```python
from build123d import *

# Parameters (mm, degrees)
BOSS_EXTRUDE1_DEPTH = 3.175
SKETCH3_R           = 1.5
CUT_EXTRUDE2_DEPTH  = 112.800002795


with BuildPart() as part:
    # Sketch1 → Boss-Extrude1 (new body)
    with BuildSketch(Plane(origin=(0, 0, 0), x_dir=(1, 0, 0), z_dir=(0, 1, 0))):
        with BuildLine():
            ThreePointArc((59, 25.4), (57.242640687, 21.157359313), (53, 19.4))
            Line((53, 19.4), (53, 17.4))
            Line((53, 17.4), (53, 17))
            Line((53, 17), (74, 17))
            Line((74, 17), (91, 17))
            ThreePointArc((91, 17), (99.746427842, 14.577379737), (106, 8))
            Line((106, 8), (106, 35.4))
            Line((106, 35.4), (53, 35.4))
            Line((53, 35.4), (53, 31.4))
            ThreePointArc((53, 31.4), (57.242640687, 29.642640687), (59, 25.4))
        make_face()
        with BuildLine():
            ThreePointArc((106, 8), (99.746427842, 14.577379737), (91, 17))
            Line((91, 17), (91, 0))
            Line((91, 0), (106, 0))
            Line((106, 0), (106, 8))
        make_face()
        with BuildLine():
            Line((91, 0), (91, 17))
            ThreePointArc((91, 17), (86.600076233, 16.420739047), (82.5, 14.722431864))
            ThreePointArc((82.5, 14.722431864), (88.722431864, 8.5), (91, 0))
        make_face()
        with BuildLine():
            Line((91, 17), (74, 17))
            ThreePointArc((74, 17), (78.399923767, 16.420739047), (82.5, 14.722431864))
            ThreePointArc((82.5, 14.722431864), (86.600076233, 16.420739047), (91, 17))
        make_face()
        with BuildLine():
            Line((53, 17.4), (53, 19.4))
            ThreePointArc((53, 19.4), (47, 25.4), (53, 31.4))
            Line((53, 31.4), (53, 35.4))
            Line((53, 35.4), (0, 35.4))
            Line((0, 35.4), (0, 8))
            ThreePointArc((0, 8), (6.253572158, 14.577379737), (15, 17))
            Line((15, 17), (32, 17))
            Line((32, 17), (53, 17))
            Line((53, 17), (53, 17.4))
        make_face()
        with BuildLine():
            Line((15, 0), (15, 17))
            ThreePointArc((15, 17), (6.253572158, 14.577379737), (0, 8))
            Line((0, 8), (0, 0))
            Line((0, 0), (15, 0))
        make_face()
        with BuildLine():
            ThreePointArc((23.5, 14.722431864), (19.399923767, 16.420739047), (15, 17))
            Line((15, 17), (15, 0))
            ThreePointArc((15, 0), (17.277568136, 8.5), (23.5, 14.722431864))
        make_face()
        with BuildLine():
            ThreePointArc((23.5, 14.722431864), (27.600076233, 16.420739047), (32, 17))
            Line((32, 17), (15, 17))
            ThreePointArc((15, 17), (19.399923767, 16.420739047), (23.5, 14.722431864))
        make_face()
    extrude(amount=BOSS_EXTRUDE1_DEPTH)

    # Sketch3 → Cut-Extrude2 (cut, through all)
    with BuildSketch(Plane.XZ):
        with BuildLine():
            ThreePointArc((9, -15), (8.560660172, -13.939339828), (7.5, -13.5))
            Line((7.5, -13.5), (7.5, -16.5))
            ThreePointArc((7.5, -16.5), (8.560660172, -16.060660172), (9, -15))
        make_face()
        with BuildLine():
            Line((7.5, -16.5), (7.5, -13.5))
            ThreePointArc((7.5, -13.5), (6, -15), (7.5, -16.5))
        make_face()
        with Locations(Location((98.5, -15, 0), (0, 0, 270))):
            Circle(SKETCH3_R)
        with Locations(Location((98.5, -7.5, 0), (0, 0, 270))):
            Circle(SKETCH3_R)
        with Locations(Location((7.5, -7.5, 0), (0, 0, 270))):
            Circle(SKETCH3_R)
    extrude(amount=-CUT_EXTRUDE2_DEPTH, mode=Mode.SUBTRACT)


solid = part.part
```
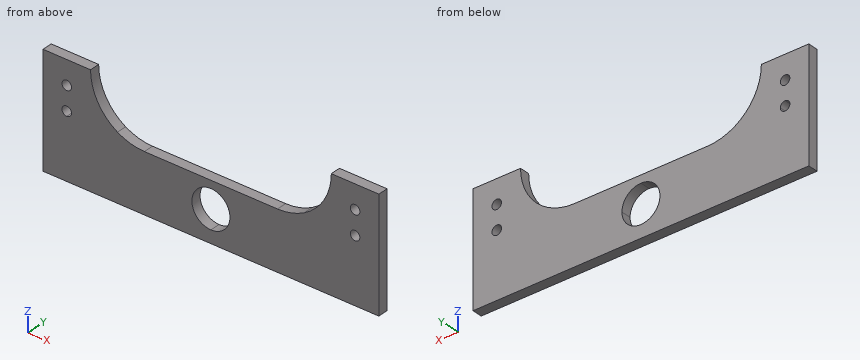
Model file for the job. Use its own axes, mm. Coordinates: 2 decimals unless noted, no trailing zeros. Write each loop counter-clockwise with the first axis right and the second up, starting at its lowest first coordinate (ties: lowest second). Pieces come first, ordered by that corner, then holes. Notation, with made-up numbers: (-23, -18) - (29, -18) arc R31 cw to (29, 8) - close; hole circle Ø6 at (10.5, -32.75). An arc over 180 degrees is marked (long way). One line per item, written item: value. Start each with the question number.
1. Slice it at B-B (z = -2). Write the cut outline in (x, y) (3 decimals), plus the area to 3 significant figures.
2. Slice it at A-A (x = 98.5). Write the cut outline in (y, z) (3 decimals).
3. Slice it at C-C (z = -7.5). Write the cut outline in (x, y) (3 decimals).
4. Slice it at D-D (x = 87.5). Write the cut outline in (y, z) (3 decimals), plus the area to 3 significant figures.
5. Probe line 1 (X direction, y = 2.15, z = -7.5); line 2 (Z direction, x = 98.5, y = 0.8); line 3 (X direction, y = 1.95, z = -15). List the from-to ranges inside material, lowest first. Write a range as from..to.
Answers below:
1. outline: (0, 0) - (15.118, 0) - (15.118, 3.175) - (0, 3.175) - close; (90.882, 0) - (106, 0) - (106, 3.175) - (90.882, 3.175) - close
1. area: 96.0 mm^2
2. outline: (0, -35.4) - (3.175, -35.4) - (3.175, -16.5) - (0, -16.5) - close; (0, -13.5) - (3.175, -13.5) - (3.175, -9) - (0, -9) - close; (0, -6) - (3.175, -6) - (3.175, 0) - (0, 0) - close
3. outline: (0, 0) - (6, 0) - (6, 3.175) - (0, 3.175) - close; (9, 0) - (16.744, 0) - (16.744, 3.175) - (9, 3.175) - close; (89.256, 0) - (97, 0) - (97, 3.175) - (89.256, 3.175) - close; (100, 0) - (106, 0) - (106, 3.175) - (100, 3.175) - close
4. outline: (0, -35.4) - (3.175, -35.4) - (3.175, -10.332) - (0, -10.332) - close
4. area: 79.6 mm^2
5. line 1: x = 0..6, 9..16.74, 89.26..97, 100..106
5. line 2: z = -35.4..-16.5, -13.5..-9, -6..0
5. line 3: x = 0..6, 9..24, 82..97, 100..106
